Part model, mm, in its own coordinate system. Face numbers are marked on the shaded views. A direction names the side the tool comes from. Coordinates: 2 decimals unless noted, no trailing zeros. Order: outer loops, then holes, each group sorted by start corner. A loop starts at its lowest first (then second) coordinate and runs counter-clockwise, first axis right, second up.
from build123d import *

# Parameters (mm, degrees)
BOSS_EXTRUDE1_DEPTH = 66
SKETCH4_R           = 15
BOSS_EXTRUDE2_DEPTH = 10
CUT_EXTRUDE2_DEPTH  = 108.615054709
SKETCH5_W           = 16
SKETCH5_H           = 23
CUT_EXTRUDE3_DEPTH  = 128.988280714
SKETCH6_W           = 10
SKETCH6_H           = 10
BOSS_EXTRUDE3_DEPTH = 5
SKETCH7_W           = 12
SKETCH7_H           = 12
BOSS_EXTRUDE4_DEPTH = 5


with BuildPart() as part:
    # Sketch2 → Boss-Extrude1 (new body)
    with BuildSketch(Plane.XY):
        with BuildLine():
            ThreePointArc((65, 0), (38.160843726, 29.198871234), (-1.89e-07, 40))
            ThreePointArc((-1.89e-07, 40), (-38.160843886, 29.198871136), (-65, 0))
            Line((-65, 0), (-65, -40))
            Line((-65, -40), (65, -40))
            Line((65, -40), (65, 0))
        make_face()
    extrude(amount=BOSS_EXTRUDE1_DEPTH)

    # Sketch4 → Boss-Extrude2 (add)
    with BuildSketch(Plane(origin=(65, 0, 0), x_dir=(0, 0, -1), z_dir=(1, 0, 0))):
        with Locations(Location((-33, -20, 0), (0, 0, 90))):
            Circle(SKETCH4_R)
    extrude(amount=BOSS_EXTRUDE2_DEPTH)

    # Sketch3 → Cut-Extrude2 (cut, through all)
    with BuildSketch(Plane.XY.offset(66)):
        with BuildLine():
            Line((-25, 5), (23, 5))
            ThreePointArc((23, 5), (30.071067812, 2.071067812), (33, -5))
            Line((33, -5), (33, -40))
            Line((33, -40), (-35, -40))
            Line((-35, -40), (-35, -5))
            ThreePointArc((-35, -5), (-32.071067812, 2.071067812), (-25, 5))
        make_face()
    extrude(amount=-CUT_EXTRUDE2_DEPTH, mode=Mode.SUBTRACT)

    # Sketch5 → Cut-Extrude3 (cut, through all)
    with BuildSketch(Plane.XZ.offset(40)):
        with Locations((-57, 54.5)):
            Rectangle(SKETCH5_W, SKETCH5_H)
        with Locations((-57, 11.5)):
            Rectangle(SKETCH5_W, SKETCH5_H)
    extrude(amount=-CUT_EXTRUDE3_DEPTH, mode=Mode.SUBTRACT)

    # Sketch6 → Boss-Extrude3 (add)
    with BuildSketch(Plane.XZ.offset(40)):
        with Locations((-48.5, 33)):
            Rectangle(SKETCH6_W, SKETCH6_H)
    extrude(amount=BOSS_EXTRUDE3_DEPTH)

    # Sketch7 → Boss-Extrude4 (add)
    with BuildSketch(Plane.XZ.offset(40)):
        with Locations((41.5, 13.9)):
            Rectangle(SKETCH7_W, SKETCH7_H)
        with Locations((41.5, 52.1)):
            Rectangle(SKETCH7_W, SKETCH7_H)
    extrude(amount=BOSS_EXTRUDE4_DEPTH)


solid = part.part
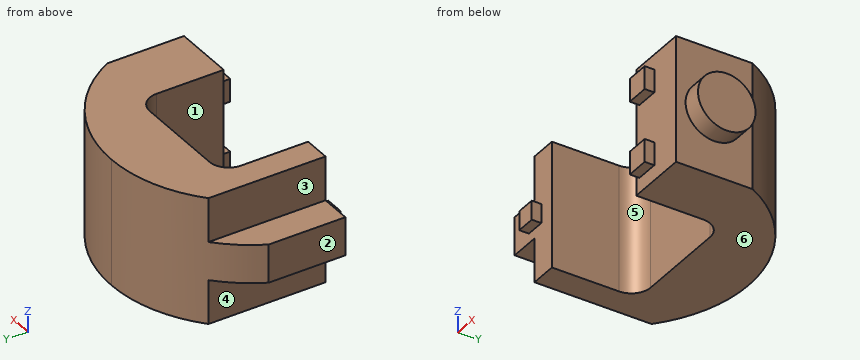
Q1. Cut at C-C on x = 46. Write the cut outline in (y, z), and give its area (3 significant figures).
Results list:
outline: (-45, 7.9) - (-40, 7.9) - (-40, 0) - (23.63, 0) - (23.63, 66) - (-40, 66) - (-40, 58.1) - (-45, 58.1) - (-45, 46.1) - (-40, 46.1) - (-40, 19.9) - (-45, 19.9) - close
area: 4,320 mm2
Q2. Which spindle directions (+Z, -Z, +X, -X, +Y, -Y) get a long thin tool onto all of the face, cutting with end or side? Do the marked faces 1, 2 and 3. Say none if no direction does.
Results list:
face 1: +Z, -Z, -Y
face 2: +Z, -Z, -X, +Y, -Y
face 3: +Z, -X, +Y, -Y
Q3. Cut at A-A on y = -20. Write the cut outline in (x, z), and give its area (3 significant figures).
Results list:
outline: (-65, 23) - (-49, 23) - (-49, 0) - (-35, 0) - (-35, 66) - (-49, 66) - (-49, 43) - (-65, 43) - close; (33, 0) - (65, 0) - (65, 18) - (75, 18) - (75, 48) - (65, 48) - (65, 66) - (33, 66) - close
area: 3,660 mm2
Q4. Cut at D-D on y = -9.5. Write the cut outline in (x, z), and give its area (3 significant figures).
Results list:
outline: (-65, 23) - (-49, 23) - (-49, 0) - (-35, 0) - (-35, 66) - (-49, 66) - (-49, 43) - (-65, 43) - close; (33, 0) - (65, 0) - (65, 22.29) - (75, 22.29) - (75, 43.71) - (65, 43.71) - (65, 66) - (33, 66) - close
area: 3,570 mm2
Q5. Pin check, flat tips, straight feed: pin 1 Ø2 at (y, z) = (14.5, 43.5) entering from -X; pin 2 Ø6 at (x, z) = (17.5, 41) entering from -Y; pin 3 Ø8 at (x, y) = (-53.5, -19) entering from -Z; pin 4 Ø5.5 at (x, y) = (41.5, -42) entering from +Z. Stop position of each tip, or through.
Results list:
pin 1: stops at x = -56.07
pin 2: stops at y = 5
pin 3: stops at z = 23
pin 4: stops at z = 66
Q6. Wall check: line 1 along X through (y, z) = (-8, 29); line 2 along X through (y, z) = (-5.5, 25.5); line 3 along Y through (x, z) = (-17, 21). Give the ranges that are in metal, low to high.
Results list:
line 1: x = -65 to -35, 33 to 75
line 2: x = -65 to -35, 33 to 65
line 3: y = 5 to 37.99
Q7. Mould opens along X. For the marked faces 4, 5 and 6 say: pulls with the +X half, pulls with the -X half, needs draft (parallel to the pull), parting line crosses it, or undercut.
Results list:
face 4: pulls with the -X half
face 5: undercut
face 6: needs draft
Q8. Cut at B-B on z = 33. Write the cut outline in (x, y) (1 decimal), and give its area (3 significant figures).
Results list:
outline: (-65, -40) - (-53.5, -40) - (-53.5, -45) - (-43.5, -45) - (-43.5, -40) - (-35, -40) - (-35, -5) arc R10 cw to (-25, 5) - (23, 5) arc R10 cw to (33, -5) - (33, -40) - (65, -40) - (65, -35) - (75, -35) - (75, -5) - (65, -5) - (65, 0) arc R72.8 ccw to (-65, 0) - close
area: 6,250 mm2
